Print and shaded views of the part. All mm, measured from the part's lowest x, y and z. A direction names the side the tool comes from. Give positions to 0.01 mm unless a question says otherwise; leave off trailing zeros. Write each loop counter-clockwise with the first axis right and the second up, starting at its lowest first coordinate (ties: lowest second). Pieces come first, ordered by that corner, then holes. Notation, with made-up numbers: (69, 73) - (76, 73) arc R25 cw to (76, 106) - close; hole circle Ø8 at (81, -30). An arc over 180 degrees is marked (long way). Use one line per item in the form item = value. Start each with the question number.
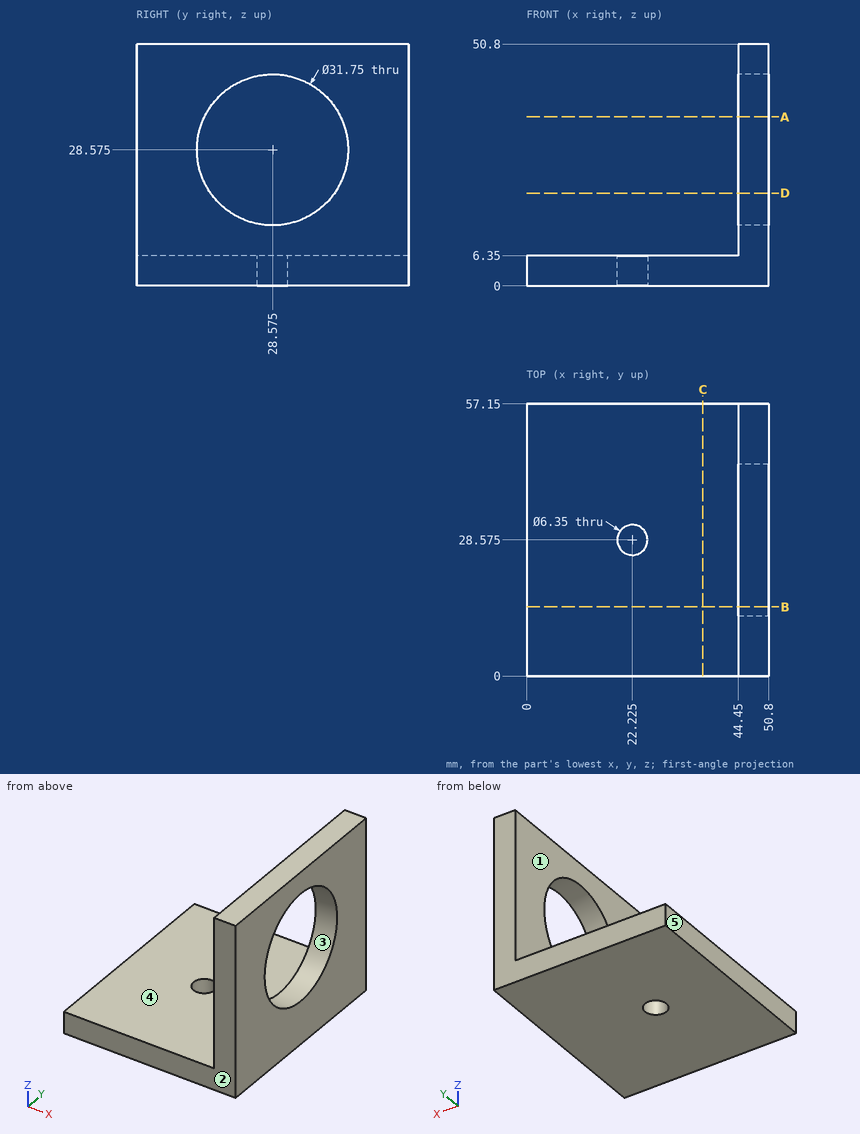
(1) Two-plate mould, pull along Y, no slides. Class the marked faces 1, 2 and 3: +Y half, -Y half, draft (parallel to the pull), parting line (faces both ways), or undercut.
(2) Cut at A-A, the plane z = 35.5. Give the cut face in (x, y).
(3) Cut at B-B, the plane y = 14.5. Give the cut face in (x, z).
(4) Which spindle directions (+Z, -Z, +X, -X, +Y, -Y) get a long thin tool onto all of the face, cutting with end or side? Do the marked faces 4 and 5. Say none if no direction does.
(5) Wall check: line 1 (Z direction, x = 31, y = 22); line 2 (X direction, y = 9, z = 33); line 3 (X direction, y = 26, z = 2). Give the ranges that are in metal, low to high. Write a range as from..to.
(6) Pin check, flat tip, straight feed: pin 1 Ø13.5 at (x, y) = (27, 29.5) entering from +Z. Stop position of the tip, or through.
(7) Cut at D-D, the plane z = 19.5. Give the cut face in (x, y), then the cut area to 3 significant figures.
(8) Cut at C-C, the plane x = 37. Give the cut face in (y, z), then the cut area to 3 significant figures.
Solution:
q1.face_1 = draft
q1.face_2 = -Y half
q1.face_3 = undercut
q2.outline = (44.45, 0) - (50.8, 0) - (50.8, 14.29) - (44.45, 14.29) - close; (44.45, 42.86) - (50.8, 42.86) - (50.8, 57.15) - (44.45, 57.15) - close
q3.outline = (0, 0) - (50.8, 0) - (50.8, 21.23) - (44.45, 21.23) - (44.45, 6.35) - (0, 6.35) - close; (44.45, 35.92) - (50.8, 35.92) - (50.8, 50.8) - (44.45, 50.8) - close
q4.face_4 = +Z, -X, +Y, -Y
q4.face_5 = +Z, -Z, -X, +Y, -Y
q5.line_1 = 0..6.35
q5.line_2 = 44.45..50.8
q5.line_3 = 0..20.37, 24.08..50.8
q6.pin_1 = 6.35
q7.outline = (44.45, 0) - (50.8, 0) - (50.8, 15.55) - (44.45, 15.55) - close; (44.45, 41.6) - (50.8, 41.6) - (50.8, 57.15) - (44.45, 57.15) - close
q7.area = 197 mm2
q8.outline = (0, 0) - (57.15, 0) - (57.15, 6.35) - (0, 6.35) - close
q8.area = 363 mm2
